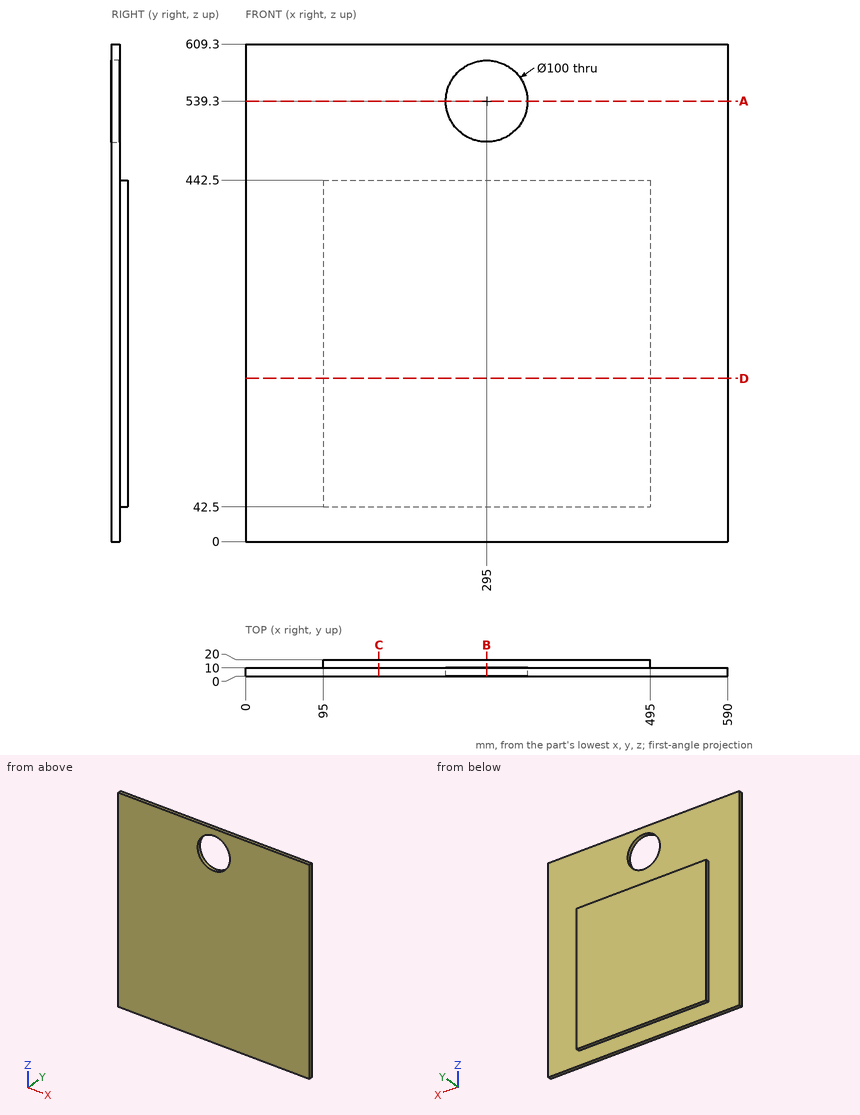
Design review of the part shown in the three views and the two pictorial views. Dimensions are in mm from the part's minimum x, y and z. Coordinates: 2 decimals unless noted, no trailing zeros. Write each loop counter-clockwise with the first axis right and the second up, starting at its lowest first coordinate (ties: lowest second). Pieces come first, ordered by that corner, then holes.
(1) Add section D-D on z = 200. Give the boundary of the cut face in (x, y), then the cut area to 3 significant figures.
(2) Wall thickness on probe 1 along X at (y, z) = (5.5, 539.3); probe 2 along X at (y, z) = (11.5, 191); probe 3 along Y at (x, z) = (125, 543): over which ranges is each line inside the solid? List them lowest first.
(3) For pin 1 Ø3 at (y, z) = (14.5, 303.5) entering from +X; pin 2 Ø5 at (x, y) = (339.5, 13.5) entering from -Z; pin 3 Ø8 at (y, z) = (16.5, 257.5) entering from -X, all flat-tipped, find the tip position at first contact; note any pin that passes through.
(4) Add section B-B on x = 295. Give the boundary of the cut face in (y, z), then the cut area to 3 significant figures.
(5) Add section A-A on z = 539.3. Give the boundary of the cut face in (x, y), then the cut area to 3 significant figures.
(6) Add section C-C on x = 163. Give the boundary of the cut face in (y, z), then the cut area to 3 significant figures.
Answer sheet:
1. outline: (0, 0) - (590, 0) - (590, 10) - (495, 10) - (495, 20) - (95, 20) - (95, 10) - (0, 10) - close
1. area: 9,900 mm2
2. probe 1: x = 0 to 245, 345 to 590
2. probe 2: x = 95 to 495
2. probe 3: y = 0 to 10
3. pin 1: stops at x = 495
3. pin 2: stops at z = 42.5
3. pin 3: stops at x = 95
4. outline: (0, 0) - (10, 0) - (10, 42.5) - (20, 42.5) - (20, 442.5) - (10, 442.5) - (10, 489.3) - (0, 489.3) - close; (0, 589.3) - (10, 589.3) - (10, 609.3) - (0, 609.3) - close
4. area: 9,090 mm2
5. outline: (0, 0) - (245, 0) - (245, 10) - (0, 10) - close; (345, 0) - (590, 0) - (590, 10) - (345, 10) - close
5. area: 4,900 mm2
6. outline: (0, 0) - (10, 0) - (10, 42.5) - (20, 42.5) - (20, 442.5) - (10, 442.5) - (10, 609.3) - (0, 609.3) - close
6. area: 10,100 mm2
